```python
from build123d import *

# Parameters (mm, degrees)
F0_W         = 10
F0_H         = 10
F1_DEPTH     = 35
F2_W         = 15
F2_H         = 15
F3_DEPTH     = 4
F4_T1_DEPTH  = 10
F4_T3_DEPTH  = 10
F4_T9_DEPTH  = 20.8253175473
F4_T14_DEPTH = 20.8253175473
F4_T22_DEPTH = 20.8253175473
F4_T27_DEPTH = 20.8253175473
F4_T35_DEPTH = 20.8253175473
F4_T40_DEPTH = 20.8253175473
F4_T48_DEPTH = 20.8253175473
F4_T53_DEPTH = 20.8253175473


# Not quite as in the source:
# - a fillet or chamfer that OpenCascade refuses, or shapes differently, is made with other operations: its cross-section is extruded or revolved along the edge and cut away or added


with BuildPart() as f1:
    # F0 (on Top) → F1 (new body)
    with BuildSketch(Plane.XY):
        Rectangle(F0_W, F0_H)
    extrude(amount=F1_DEPTH)

    # F2 (on Top) → F3 (join)
    with BuildSketch(Plane.XY):
        Rectangle(F2_W, F2_H)
    extrude(amount=F3_DEPTH)

    # F4: fillet of radius 5 on 4 edges, made by hand

    # F4_s2 → F4_t1 (join)
    with BuildSketch(Plane.XZ.offset(-5)):
        with BuildLine():
            ThreePointArc((-7.5, 4), (-5.6698729811, 5.8301270189), (-5, 8.3301270189))
            Line((-5, 8.3301270189), (-5, 4))
            Line((-5, 4), (-7.5, 4))
        make_face()
        with BuildLine():
            ThreePointArc((7.5, 4), (5.6698729811, 5.8301270189), (5, 8.3301270189))
            Line((5, 8.3301270189), (5, 4))
            Line((5, 4), (7.5, 4))
        make_face()
    extrude(amount=F4_T1_DEPTH)

    # F4_s4 → F4_t3 (join)
    with BuildSketch(Plane.YZ.offset(-5)):
        with BuildLine():
            ThreePointArc((7.5, 4), (5.6698729811, 5.8301270189), (5, 8.3301270189))
            Line((5, 8.3301270189), (5, 4))
            Line((5, 4), (7.5, 4))
        make_face()
        with BuildLine():
            ThreePointArc((-7.5, 4), (-5.6698729811, 5.8301270189), (-5, 8.3301270189))
            Line((-5, 8.3301270189), (-5, 4))
            Line((-5, 4), (-7.5, 4))
        make_face()
    extrude(amount=F4_T3_DEPTH)


with BuildPart() as f4_tool7:
    # F4_s8 → F4_t9 (new body)
    with BuildSketch(Plane.YZ.offset(5)):
        with BuildLine():
            ThreePointArc((7.5, 4), (5.6698729811, 5.8301270189), (5, 8.3301270189))
            Line((5, 8.3301270189), (5, 4))
            Line((5, 4), (7.5, 4))
        make_face()
    extrude(amount=-F4_T9_DEPTH)

    split(bisect_by=Plane.YZ.offset(-7.5), keep=Keep.TOP)

    split(bisect_by=Plane.YZ.offset(-5), keep=Keep.BOTTOM)


with BuildPart() as f4_tool12:
    # F4_s13 → F4_t14 (new body)
    with BuildSketch(Plane.XZ.offset(-15.8253175473)):
        with BuildLine():
            ThreePointArc((-7.5, 4), (-5.6698729811, 5.8301270189), (-5, 8.3301270189))
            Line((-5, 8.3301270189), (-5, 4))
            Line((-5, 4), (-7.5, 4))
        make_face()
    extrude(amount=F4_T14_DEPTH)

    split(bisect_by=Plane.XZ.offset(-7.5), keep=Keep.TOP)

    split(bisect_by=Plane.XZ.offset(-5), keep=Keep.BOTTOM)


with BuildPart() as f4_tool7_1:
    add(f4_tool7.part)

    # F4_t17: intersect F4_tool12
    add(f4_tool12.part, mode=Mode.INTERSECT)


with BuildPart() as f1_1:
    add(f1.part)

    # F4_t5: union F4_tool7
    add(f4_tool7_1.part)


with BuildPart() as f4_tool20:
    # F4_s21 → F4_t22 (new body)
    with BuildSketch(Plane.XZ.offset(-5)):
        with BuildLine():
            ThreePointArc((-7.5, 4), (-5.6698729811, 5.8301270189), (-5, 8.3301270189))
            Line((-5, 8.3301270189), (-5, 4))
            Line((-5, 4), (-7.5, 4))
        make_face()
    extrude(amount=F4_T22_DEPTH)

    split(bisect_by=Plane.XZ.offset(7.5), keep=Keep.BOTTOM)

    split(bisect_by=Plane.XZ.offset(5), keep=Keep.TOP)


with BuildPart() as f4_tool25:
    # F4_s26 → F4_t27 (new body)
    with BuildSketch(Plane.YZ.offset(-15.8253175473)):
        with BuildLine():
            ThreePointArc((-7.5, 4), (-5.6698729811, 5.8301270189), (-5, 8.3301270189))
            Line((-5, 8.3301270189), (-5, 4))
            Line((-5, 4), (-7.5, 4))
        make_face()
    extrude(amount=F4_T27_DEPTH)

    split(bisect_by=Plane.YZ.offset(-7.5), keep=Keep.TOP)

    split(bisect_by=Plane.YZ.offset(-5), keep=Keep.BOTTOM)


with BuildPart() as f4_tool20_1:
    add(f4_tool20.part)

    # F4_t30: intersect F4_tool25
    add(f4_tool25.part, mode=Mode.INTERSECT)


with BuildPart() as f1_2:
    add(f1_1.part)

    # F4_t18: union F4_tool20
    add(f4_tool20_1.part)


with BuildPart() as f4_tool33:
    # F4_s34 → F4_t35 (new body)
    with BuildSketch(Plane.YZ.offset(15.8253175473)):
        with BuildLine():
            ThreePointArc((7.5, 4), (5.6698729811, 5.8301270189), (5, 8.3301270189))
            Line((5, 8.3301270189), (5, 4))
            Line((5, 4), (7.5, 4))
        make_face()
    extrude(amount=-F4_T35_DEPTH)

    split(bisect_by=Plane.YZ.offset(7.5), keep=Keep.BOTTOM)

    split(bisect_by=Plane.YZ.offset(5), keep=Keep.TOP)


with BuildPart() as f4_tool38:
    # F4_s39 → F4_t40 (new body)
    with BuildSketch(Plane.XZ.offset(5)):
        with BuildLine():
            ThreePointArc((7.5, 4), (5.6698729811, 5.8301270189), (5, 8.3301270189))
            Line((5, 8.3301270189), (5, 4))
            Line((5, 4), (7.5, 4))
        make_face()
    extrude(amount=-F4_T40_DEPTH)

    split(bisect_by=Plane.XZ.offset(-7.5), keep=Keep.TOP)

    split(bisect_by=Plane.XZ.offset(-5), keep=Keep.BOTTOM)


with BuildPart() as f4_tool33_1:
    add(f4_tool33.part)

    # F4_t43: intersect F4_tool38
    add(f4_tool38.part, mode=Mode.INTERSECT)


with BuildPart() as f1_3:
    add(f1_2.part)

    # F4_t31: union F4_tool33
    add(f4_tool33_1.part)


with BuildPart() as f4_tool46:
    # F4_s47 → F4_t48 (new body)
    with BuildSketch(Plane.YZ.offset(-5)):
        with BuildLine():
            ThreePointArc((-7.5, 4), (-5.6698729811, 5.8301270189), (-5, 8.3301270189))
            Line((-5, 8.3301270189), (-5, 4))
            Line((-5, 4), (-7.5, 4))
        make_face()
    extrude(amount=F4_T48_DEPTH)

    split(bisect_by=Plane.YZ.offset(7.5), keep=Keep.BOTTOM)

    split(bisect_by=Plane.YZ.offset(5), keep=Keep.TOP)


with BuildPart() as f4_tool51:
    # F4_s52 → F4_t53 (new body)
    with BuildSketch(Plane.XZ.offset(15.8253175473)):
        with BuildLine():
            ThreePointArc((7.5, 4), (5.6698729811, 5.8301270189), (5, 8.3301270189))
            Line((5, 8.3301270189), (5, 4))
            Line((5, 4), (7.5, 4))
        make_face()
    extrude(amount=-F4_T53_DEPTH)

    split(bisect_by=Plane.XZ.offset(7.5), keep=Keep.BOTTOM)

    split(bisect_by=Plane.XZ.offset(5), keep=Keep.TOP)


with BuildPart() as f4_tool46_1:
    add(f4_tool46.part)

    # F4_t56: intersect F4_tool51
    add(f4_tool51.part, mode=Mode.INTERSECT)


with BuildPart() as f1_4:
    add(f1_3.part)

    # F4_t44: union F4_tool46
    add(f4_tool46_1.part)


solid = f1_4.part
```
Could you check a few things on this model? Use its own coordinates, in mm. A direction names the side the tool comes from. Round coordinates to 2 decimals unless told otherwise and drop trailing zeros. Loops run counter-clockwise (first coordinate to the right, second up) from the corner with the lowest first, then second, coordinate; pieces in that order, holes last. Notation, with made-up numbers: (-23.75, -12) - (32.25, -12) arc R27 ccw to (32.25, 26) - close; hole circle Ø9 at (-20, 58). An arc over 180 degrees is marked (long way). Answer in a Markdown table with one row per item. Add a question column.
(1) I'm going to push flat-ended pins straight in: pin 1 (8 mm diameter, centred on y = 1.5, z = 16, fed in from -X); pin 2 (3 mm diameter, centred on x = 1.5, z = 17.5, fed in from -Y); pin 3 (8 mm diameter, centred on y = -4.5, z = 23.5, fed in from +X). Where does each tip first touch, or does it pass through?
(2) For faces 1 (the face through (-5, 0, 21)), 2 (the face through (0, 5, 22)), 3 (the face through (0, 0, 35)), 4 (the face through (5, 0, 21)), 5 (the face through (0, -5, 22)), which set-ups out of +Z, -Z, +X, -X, +Y, -Y let a thin tool reach every point of the face, with its end or its side?
(3) I need wall thicknesses on line 1 along X through (y, z) = (-3.25, 26.5); line 2 along Z through (x, y) = (-2.75, 6.5). Which ranges of each line are inside material? Lowest first, please.
(4) If we section it at C-C (z = 19.5): Please give me the cut outline in (x, y), plus the area to 3 significant figures.
(5) If we section it at D-D (x = -5.5): Please give me the cut outline in (y, z), plus the area to 3 significant figures.
(6) If we section it at A-A (y = 3.5): Please give me the cut outline in (x, z), plus the area to 3 significant figures.
Model answer:
| question | item | result |
|---|---|---|
| 1 | pin 1 | stops at x = -5 |
| 1 | pin 2 | stops at y = -5 |
| 1 | pin 3 | stops at x = 5 |
| 2 | face 1 | +Z, -X, +Y, -Y |
| 2 | face 2 | +Z, +X, -X, +Y |
| 2 | face 3 | +Z, +X, -X, +Y, -Y |
| 2 | face 4 | +Z, +X, +Y, -Y |
| 2 | face 5 | +Z, +X, -X, -Y |
| 3 | line 1 | x = -5 to 5 |
| 3 | line 2 | z = 0 to 4.76 |
| 4 | outline | (-5, -5) - (5, -5) - (5, 5) - (-5, 5) - close |
| 4 | area | 100 mm² |
| 5 | outline | (-7.5, 0) - (7.5, 0) - (7.5, 4) arc R5 cw to (5.5, 6.15) - (-5.5, 6.15) arc R5 cw to (-7.5, 4) - close |
| 5 | area | 87.1 mm² |
| 6 | outline | (-7.5, 0) - (7.5, 0) - (7.5, 4) arc R5 cw to (5, 8.33) - (5, 35) - (-5, 35) - (-5, 8.33) arc R5 cw to (-7.5, 4) - close |
| 6 | area | 376 mm² |
